from build123d import *

# Parameters (mm, degrees)
BOSS_EXTRUDE1_DEPTH            = 32.5
SKETCH2_W                      = 32.5
SKETCH2_H                      = 25.708203932
BOSS_EXTRUDE2_DEPTH            = 8
CUT_EXTRUDE1_DEPTH             = 17.032
SKETCH4_W                      = 32.5
SKETCH4_H                      = 8
BOSS_EXTRUDE3_DEPTH            = 7
SKETCH5_W                      = 7.734
SKETCH5_H                      = 11
BOSS_EXTRUDE4_DEPTH            = 29.291796068
SKETCH6_W                      = 7.734
SKETCH6_H                      = 11
BOSS_EXTRUDE5_DEPTH            = 29.291796068
SKETCH7_W                      = 17.032
SKETCH7_H                      = 30
BOSS_EXTRUDE6_DEPTH            = 6
CUT_EXTRUDE3_REACH             = 75.331
CUT_EXTRUDE4_DEPTH             = 6.5
CUT_EXTRUDE5_DEPTH             = 4
SKETCH12_W                     = 4.2
SKETCH12_H                     = 8.5
CUT_EXTRUDE6_DEPTH             = 12.5
SKETCH13_W                     = 4.2
SKETCH13_H                     = 8.5
CUT_EXTRUDE7_DEPTH             = 12.5
F_5_1_5_1_DIAMETER_HOLE1_D     = 5.1
F_5_1_5_1_DIAMETER_HOLE1_DEPTH = 2
F_5_1_5_1_DIAMETER_HOLE2_D     = 5.1
F_5_1_5_1_DIAMETER_HOLE2_DEPTH = 2
F_6_0_6_DIAMETER_HOLE1_D       = 6
F_6_0_6_DIAMETER_HOLE1_DEPTH   = 7.73405
HOLE1_D                        = 6
HOLE1_DEPTH                    = 32.50005
HOLE1_CBORE_D                  = 9.5
HOLE1_CBORE_DEPTH              = 6.5
F_6_0_6_DIAMETER_HOLE2_D       = 6
F_5_1_5_1_DIAMETER_HOLE3_D     = 5.1
F_5_1_5_1_DIAMETER_HOLE3_DEPTH = 26.30005
FILLET1_R                      = 2.5
FILLET2_R                      = 5


with BuildPart() as part:
    # Sketch1 → Boss-Extrude1 (new body)
    with BuildSketch(Plane(origin=(31.766, 0, 0), x_dir=(0, 0, -1), z_dir=(1, 0, 0))):
        with BuildLine():
            Line((-14, 26), (-14, 32.708203932))
            Line((-14, 32.708203932), (-17, 32.708203932))
            ThreePointArc((-17, 32.708203932), (-16.215838363, 29.033969318), (-14, 26))
        make_face()
    extrude(amount=-BOSS_EXTRUDE1_DEPTH)

    # Sketch2 → Boss-Extrude2 (add)
    with BuildSketch(Plane(origin=(0, 0, 14), x_dir=(-1, 0, 0), z_dir=(0, 0, -1))):
        with Locations((-15.516, 19.854101966)):
            Rectangle(SKETCH2_W, SKETCH2_H)
    extrude(amount=BOSS_EXTRUDE2_DEPTH)

    # Sketch3 → Cut-Extrude1 (cut)
    with BuildSketch(Plane(origin=(24.032, 0, 0), x_dir=(0, 0, -1), z_dir=(1, 0, 0))):
        with BuildLine():
            Line((-6, 15), (-6, 32.708203932))
            Line((-6, 32.708203932), (-17, 32.708203932))
            ThreePointArc((-17, 32.708203932), (-16.215838363, 29.033969318), (-14, 26))
            Line((-14, 26), (-14, 7))
            ThreePointArc((-14, 7), (-11.656854249, 12.656854249), (-6, 15))
        make_face()
    extrude(amount=-CUT_EXTRUDE1_DEPTH, mode=Mode.SUBTRACT)

    # Sketch4 → Boss-Extrude3 (add)
    with BuildSketch(Plane.XZ.offset(-7)):
        with Locations((15.516, 10)):
            Rectangle(SKETCH4_W, SKETCH4_H)
    extrude(amount=BOSS_EXTRUDE3_DEPTH)

    # Sketch5 → Boss-Extrude4 (add)
    with BuildSketch(Plane(origin=(0, 32.708203932, 0), x_dir=(-1, 0, 0), z_dir=(0, 1, 0))):
        with Locations((-27.899, 11.5)):
            Rectangle(SKETCH5_W, SKETCH5_H)
    extrude(amount=BOSS_EXTRUDE4_DEPTH)

    # Sketch6 → Boss-Extrude5 (add)
    with BuildSketch(Plane(origin=(0, 32.708203932, 0), x_dir=(-1, 0, 0), z_dir=(0, 1, 0))):
        with Locations((-3.133, 11.5)):
            Rectangle(SKETCH6_W, SKETCH6_H)
    extrude(amount=BOSS_EXTRUDE5_DEPTH)

    # Sketch7 → Boss-Extrude6 (add)
    with BuildSketch(Plane(origin=(0, 0, 6), x_dir=(-1, 0, 0), z_dir=(0, 0, -1))):
        with BuildLine():
            Line((0.734, 62), (0.734, 0))
            Line((0.734, 0), (-31.766, 0))
            Line((-31.766, 0), (-31.766, 62))
            Line((-31.766, 62), (-19.669311931, 62))
            ThreePointArc((-19.669311931, 62), (-15.516, 63.5), (-11.362688069, 62))
            Line((-11.362688069, 62), (0.734, 62))
        make_face()
        with Locations((-15.516, 35)):
            Rectangle(SKETCH7_W, SKETCH7_H, mode=Mode.SUBTRACT)
    extrude(amount=BOSS_EXTRUDE6_DEPTH)

    # Cut-Extrude3: up to this face of the body (flat: up to its plane)
    cut_extrude3_end = Plane(part.part.faces().sort_by_distance((-0.734, 32.469284898, 7.888317221))[0])
    # Sketch9 → Cut-Extrude3 (cut, up to the picked face)
    with BuildSketch(Plane(origin=(31.766, 0, 0), x_dir=(0, 0, -1), z_dir=(1, 0, 0)), mode=Mode.PRIVATE) as cut_extrude3_sk1:
        with BuildLine():
            Line((-11, 43.520866203), (-11, 62))
            Line((-11, 62), (-17, 62))
            Line((-17, 62), (-17, 35))
            ThreePointArc((-17, 35), (-15.5, 39.974937186), (-11.5, 43.291561976))
            ThreePointArc((-11.5, 43.291561976), (-11.248247728, 43.402393245), (-11, 43.520866203))
        make_face()
    cut_extrude3_tool1 = split(extrude(cut_extrude3_sk1.sketch, amount=-CUT_EXTRUDE3_REACH, mode=Mode.PRIVATE), bisect_by=cut_extrude3_end, keep=Keep.BOTH, mode=Mode.PRIVATE)
    add(cut_extrude3_tool1.solids().sort_by(Axis((31.766, 51.50501, 14.153169), (-1, 0, 0)))[0], mode=Mode.SUBTRACT)

    # Sketch10 → Cut-Extrude4 (cut)
    with BuildSketch(Plane.ZY.offset(0.734)):
        Polygon((8.5, 40.051814855), (4.125, 37.525907428), (4.125, 32.474092572), (8.5, 29.948185145), (12.875, 32.474092572), (12.875, 37.525907428), align=None)
    extrude(amount=-CUT_EXTRUDE4_DEPTH, mode=Mode.SUBTRACT)

    # Sketch11 → Cut-Extrude5 (cut)
    with BuildSketch(Plane(origin=(0, 0, 0), x_dir=(-1, 0, 0), z_dir=(0, 0, -1))):
        Polygon((-17.835622857, 61.1), (-20.202758961, 57), (-17.835622857, 52.9), (-13.10135065, 52.9), (-10.734214546, 57), (-13.10135065, 61.1), align=None)
    extrude(amount=-CUT_EXTRUDE5_DEPTH, mode=Mode.SUBTRACT)

    # Sketch12 → Cut-Extrude6 (cut)
    with BuildSketch(Plane.XZ):
        with Locations((27.666, 7.5)):
            Rectangle(SKETCH12_W, SKETCH12_H)
    extrude(amount=-CUT_EXTRUDE6_DEPTH, mode=Mode.SUBTRACT)

    # Sketch13 → Cut-Extrude7 (cut)
    with BuildSketch(Plane.XZ):
        with Locations((3.366, 7.5)):
            Rectangle(SKETCH13_W, SKETCH13_H)
    extrude(amount=-CUT_EXTRUDE7_DEPTH, mode=Mode.SUBTRACT)

    # Ø5.1 (5.1) Diameter Hole1
    with Locations(Plane(origin=(31.766, 0, 0), x_dir=(0, 0, -1), z_dir=(1, 0, 0))):
        with Locations((-7.5, 6)):
            Hole(F_5_1_5_1_DIAMETER_HOLE1_D / 2, depth=F_5_1_5_1_DIAMETER_HOLE1_DEPTH)

    # Ø5.1 (5.1) Diameter Hole2
    with Locations(Plane.ZY.offset(0.734)):
        with Locations((7.5, 6)):
            Hole(F_5_1_5_1_DIAMETER_HOLE2_D / 2, depth=F_5_1_5_1_DIAMETER_HOLE2_DEPTH)

    # Ø6.0 (6) Diameter Hole1
    with Locations(Plane(origin=(7, 0, 0), x_dir=(0, 0, -1), z_dir=(1, 0, 0))):
        with Locations((-8.5, 35)):
            Hole(F_6_0_6_DIAMETER_HOLE1_D / 2, depth=F_6_0_6_DIAMETER_HOLE1_DEPTH)

    # Hole1
    with Locations(Plane(origin=(31.766, 0, 0), x_dir=(0, 0, -1), z_dir=(1, 0, 0))):
        with Locations((-8.5, 35)):
            CounterBoreHole(HOLE1_D / 2, HOLE1_CBORE_D / 2, HOLE1_CBORE_DEPTH, depth=HOLE1_DEPTH)

    # Ø6.0 (6) Diameter Hole2 (through all)
    with Locations(Plane.XY.offset(6)):
        with Locations((15.516, 57)):
            Hole(F_6_0_6_DIAMETER_HOLE2_D / 2)

    # Ø5.1 (5.1) Diameter Hole3
    with Locations(Plane.ZY.offset(-5.466)):
        with Locations((7.5, 6)):
            Hole(F_5_1_5_1_DIAMETER_HOLE3_D / 2, depth=F_5_1_5_1_DIAMETER_HOLE3_DEPTH)

    # Fillet1
    fillet1_edges = [part.edges().sort_by_distance(p)[0] for p in [
        (7, 20, 3),
        (24.032, 20, 3),
        (7, 50, 3),
        (24.032, 50, 3),
    ]]
    fillet(fillet1_edges, radius=FILLET1_R)

    # Fillet2
    # the kernel refuses this fillet: 5 mm, written as the material it adds along each edge
    with BuildSketch(Plane(origin=(34.032, 15, 6), x_dir=(0, 1, 0), z_dir=(-1, 0, 0))) as fillet2_piece_1_section:
        with BuildLine():
            CenterArc((4, -5), FILLET2_R, 90, 67.380135052)
            ThreePointArc((-0.615384615, -3.076923077), (-0.155354594, -1.568929081), (0, 0))
            Line((0, 0), (4, 0))
        make_face()
    fillet2_piece_1 = extrude(amount=27.032, mode=Mode.PRIVATE)
    fillet2_piece_1 = split(fillet2_piece_1, bisect_by=Plane(origin=(31.766, 15.849865024, 6.687390225), z_dir=(-1, 0, 0)), keep=Keep.TOP, mode=Mode.PRIVATE)
    add(fillet2_piece_1)
    # the kernel refuses this fillet: 5 mm, written as the material it takes off along each edge
    with BuildSketch(Plane(origin=(-0.734, 62, 23.5), x_dir=(1, 0, 0), z_dir=(0, 0, -1)), Plane(origin=(31.766, 62, -12.5), x_dir=(-1, 0, 0), z_dir=(0, 0, 1))) as fillet2_2_piece_1:
        with BuildLine():
            CenterArc((FILLET2_R, FILLET2_R), FILLET2_R, 180, 90)
            Line((0, FILLET2_R), (0, 0))
            Line((0, 0), (FILLET2_R, 0))
        make_face()
    extrude(amount=36, mode=Mode.SUBTRACT)
    with BuildSketch(Plane(origin=(-13.234, 0, 0), x_dir=(0, 1, 0), z_dir=(1, 0, 0))) as fillet2_2_piece_2:
        with BuildLine():
            CenterArc((FILLET2_R, FILLET2_R), FILLET2_R, 180, 90)
            Line((0, FILLET2_R), (0, 0))
            Line((0, 0), (FILLET2_R, 0))
        make_face()
    extrude(amount=57.5, mode=Mode.SUBTRACT)
    with BuildSketch(Plane(origin=(44.266, 62, 11), x_dir=(0, -1, 0), z_dir=(-1, 0, 0))) as fillet2_2_piece_3:
        with BuildLine():
            CenterArc((FILLET2_R, -FILLET2_R), FILLET2_R, 90, 90)
            Line((0, -FILLET2_R), (0, 0))
            Line((0, 0), (FILLET2_R, 0))
        make_face()
    extrude(amount=32.734, mode=Mode.SUBTRACT)
    with BuildSketch(Plane(origin=(-13.234, 0, 14), x_dir=(0, 1, 0), z_dir=(1, 0, 0))) as fillet2_2_piece_4:
        with BuildLine():
            CenterArc((FILLET2_R, -FILLET2_R), FILLET2_R, 90, 90)
            Line((0, -FILLET2_R), (0, 0))
            Line((0, 0), (FILLET2_R, 0))
        make_face()
    extrude(amount=57.5, mode=Mode.SUBTRACT)
    with BuildSketch(Plane(origin=(19.5, 62, 11), x_dir=(0, 0, -1), z_dir=(-1, 0, 0))) as fillet2_2_piece_5:
        with BuildLine():
            CenterArc((FILLET2_R, FILLET2_R), FILLET2_R, 180, 90)
            Line((0, FILLET2_R), (0, 0))
            Line((0, 0), (FILLET2_R, 0))
        make_face()
    extrude(amount=32.734, mode=Mode.SUBTRACT)


solid = part.part
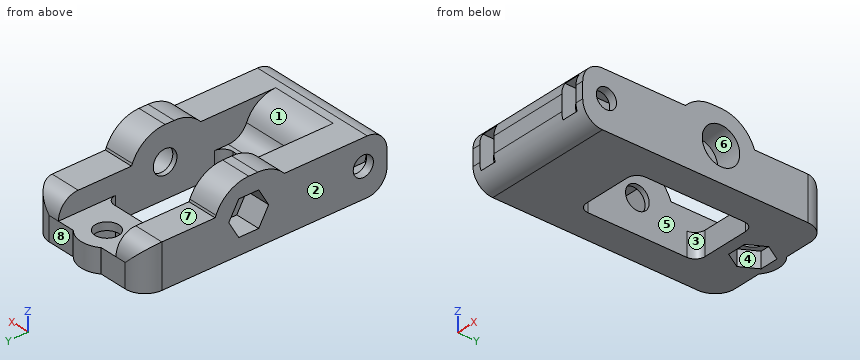
Can you work these out from the model? Positions are in its coordinate system, mm. Face numbers are marked on the shaded views. A direction names the side the tool comes from. Give positions to 0.01 mm unless a question says otherwise; leave off trailing zeros. Order: outer loops, then holes, each group sorted by start corner. A loop starts at its lowest first (then second) coordinate and runs counter-clockwise, first axis right, second up. Notation, with made-up numbers: M 70,-38 L 89,-38 A5 ccw 89,-31 Z; hole C 31.5,5.5 d4. An arc over 180 degrees is marked long. One line per question, with ' | ' between items.
Item 1: For the marked faces 5, 6, 7 and 8, which set-ups out of +Z, -Z, +X, -X, +Y, -Y let a thin tool reach every point of the face, with its end or its side?
Answer block:
face 5: +Z | face 6: +X | face 7: +Z, +X, -X, +Y | face 8: +Z, -Z, +X, +Y
Item 2: Suppose I cut it at D-D, the plane y = 45. Write out the boundary of the cut face in (x, z).
Answer block:
outline: M -0.73,0 L 7,0 L 7,11 L -0.73,11 Z; M 24.03,0 L 31.77,0 L 31.77,11 L 24.03,11 Z
Item 3: Please list where these lines run through material, in increasing order: L1, parallel to X at y = 20, z = 7; L2, parallel to Y at x = -0.3, z = 7.5; L3, parallel to Y at x = 25, z = 9.
Answer block:
L1: x = -0.73 to 7, 24.03 to 31.77 | L2: y = 0 to 3.45, 8.55 to 30.53, 39.47 to 59.04 | L3: y = 0 to 3.94, 8.06 to 32.04, 37.96 to 61
Item 4: We'd pull the mould along Y, two halves only. Please class the marked faces 1, 2, 3 and 4: released by +Y, released by -Y, zero draft, split by the parting line, or undercut.
Answer block:
face 1: released by +Y | face 2: zero draft | face 3: undercut | face 4: undercut
Item 5: I'm going to push flat-ended pins straight in: pin 1 Ø1.8 at (x, z) = (17, 3.5) entering from -Y; pin 2 Ø10.5 at (x, y) = (19, 13.5) entering from +Z; pin 3 Ø2 at (x, y) = (10, 7.5) entering from -Z; pin 4 Ø3 at (x, z) = (24, 3.5) entering from +Y. Where does each tip first touch, or does it pass through?
Answer block:
pin 1: stops at y = 0.04 | pin 2: stops at z = 14 | pin 3: stops at z = 0 | pin 4: stops at y = 62
Item 6: Suppose I cut it at C-C, the plane z = 2.25. Write out the boundary of the cut face in (x, y).
Answer block:
outline: M -0.73,0.82 L 31.77,0.82 L 31.77,57 A5 ccw 26.77,62 L 19.67,62 A6.5 ccw 11.36,62 L 4.27,62 A5 ccw -0.73,57 Z; hole M 7,22.5 A2.5 ccw 9.5,20 L 21.53,20 A2.5 ccw 24.03,22.5 L 24.03,47.5 A2.5 ccw 21.53,50 L 9.5,50 A2.5 ccw 7,47.5 Z; hole M 10.73,57 L 13.1,52.9 L 17.84,52.9 L 20.2,57 L 17.84,61.1 L 13.1,61.1 Z
Item 7: Suppose I cut it at A-A, the plane y = 6. Write out the boundary of the cut face in (x, z), then the cut area to 3 significant figures.
Answer block:
outline: M -0.73,0 L 31.77,0 L 31.77,4.95 L 29.77,4.95 L 29.77,3.25 L 25.57,3.25 L 25.57,4.95 L 5.47,4.95 L 5.47,3.25 L 1.27,3.25 L 1.27,4.95 L -0.73,4.95 Z; M -0.73,10.05 L 1.27,10.05 L 1.27,11.75 L 5.47,11.75 L 5.47,10.05 L 25.57,10.05 L 25.57,11.75 L 29.77,11.75 L 29.77,10.05 L 31.77,10.05 L 31.77,14 L -0.73,14 Z | area: 261 mm2
Item 8: Suppose I cut it at B-B, the plane x = 16.5. Write out the boundary of the cut face in (y, z).
Answer block:
outline: M 0,5 A5 ccw 5,0 L 20,0 L 20,6 L 19,6 A5 cw 14.38,9.08 A8 ccw 7,14 L 5,14 A5 ccw 0,9 Z; M 50,0 L 52.9,0 L 52.9,4 L 54.17,4 L 54.17,6 L 50,6 Z; M 59.83,4 L 61.1,4 L 61.1,0 L 63.43,0 L 63.43,6 L 59.83,6 Z; hole C 6,7.5 d5.1
